Check sheet for the modelled part. Datum: model origin and axes. Units: mm. Round coordinates to 2 decimals unless told otherwise and drop trailing zeros. Order: outer loops, then holes, each group sorted by start corner. A loop starts at its lowest first (then second) coordinate and runs counter-clockwise, first axis right, second up.
```python
from build123d import *

# Parameters (mm, degrees)
F1_DEPTH = 38.1
F2_DEPTH = 38.1
F4_DEPTH = 38.1
F5_DEPTH = 38.1
F7_DEPTH = 38.1
F8_DEPTH = 38.1


with BuildPart() as f1:
    # F0 (on Front) → F1 (new body)
    with BuildSketch(Plane.XZ):
        Polygon((-19.05, 38.1), (-38.1, 19.05), (-38.1, -19.05), (-19.05, -38.1), (19.05, -38.1), (38.1, -19.05), (38.1, 19.05), (19.05, 38.1), align=None)
    extrude(amount=F1_DEPTH)

    # F0 (on Front) → F2 (join)
    with BuildSketch(Plane.XZ):
        Polygon((-19.05, 38.1), (-38.1, 19.05), (-38.1, -19.05), (-19.05, -38.1), (19.05, -38.1), (38.1, -19.05), (38.1, 19.05), (19.05, 38.1), align=None)
    extrude(amount=-F2_DEPTH)

    # F3 (on Right) → F4 (cut)
    with BuildSketch(Plane.YZ):
        Polygon((-38.1, 38.1), (-38.1, 19.05), (-19.05, 38.1), align=None)
        Polygon((38.1, 38.1), (19.05, 38.1), (38.1, 19.05), align=None)
        Polygon((38.1, -19.05), (19.05, -38.1), (38.1, -38.1), align=None)
        Polygon((-19.05, -38.1), (-38.1, -19.05), (-38.1, -38.1), align=None)
    extrude(amount=-F4_DEPTH, mode=Mode.SUBTRACT)

    # F3 (on Right) → F5 (cut)
    with BuildSketch(Plane.YZ):
        Polygon((-38.1, 38.1), (-38.1, 19.05), (-19.05, 38.1), align=None)
        Polygon((38.1, 38.1), (19.05, 38.1), (38.1, 19.05), align=None)
        Polygon((38.1, -19.05), (19.05, -38.1), (38.1, -38.1), align=None)
        Polygon((-19.05, -38.1), (-38.1, -19.05), (-38.1, -38.1), align=None)
    extrude(amount=F5_DEPTH, mode=Mode.SUBTRACT)

    # F6 (on Top) → F7 (cut)
    with BuildSketch(Plane.XY):
        Polygon((38.1, -19.05), (19.05, -38.1), (38.1, -38.1), align=None)
        Polygon((19.05, 38.1), (38.1, 19.05), (38.1, 38.1), align=None)
        Polygon((-38.1, 38.1), (-38.1, 19.05), (-19.05, 38.1), align=None)
        Polygon((-38.1, -38.1), (-19.05, -38.1), (-38.1, -19.05), align=None)
    extrude(amount=-F7_DEPTH, mode=Mode.SUBTRACT)

    # F6 (on Top) → F8 (cut)
    with BuildSketch(Plane.XY):
        Polygon((38.1, -19.05), (19.05, -38.1), (38.1, -38.1), align=None)
        Polygon((-38.1, -38.1), (-19.05, -38.1), (-38.1, -19.05), align=None)
        Polygon((-38.1, 38.1), (-38.1, 19.05), (-19.05, 38.1), align=None)
        Polygon((19.05, 38.1), (38.1, 19.05), (38.1, 38.1), align=None)
    extrude(amount=F8_DEPTH, mode=Mode.SUBTRACT)


solid = f1.part
```
Item 1: Scan lines: line 1 along Z through (x, y) = (28.5, -9); line 2 along Z through (x, y) = (-20.5, 24); line 3 along X through (y, z) = (21, 34). Record each from-to range of solid material in increasing order.
Answer:
line 1: z = -28.65 to 28.65
line 2: z = -33.15 to 33.15
line 3: x = -23.15 to 23.15
Item 2: Sectioned sample at B-B (y = -25.5). Record the cut outline in (x, z), and give its area (3 significant figures).
Answer:
outline: (-31.65, -25.5) - (-25.5, -31.65) - (25.5, -31.65) - (31.65, -25.5) - (31.65, 25.5) - (25.5, 31.65) - (-25.5, 31.65) - (-31.65, 25.5) - close
area: 3,930 mm2
Item 3: Go/stop test with flat-tipped pins: P1, Ø10, axis at x = 30.5, z = 7, coming from the +Y side; P2, Ø1, axis at x = -20.5, y = -14.5, coming from the -Z side; P3, Ø4, axis at x = -30, z = 11, coming from the +Y side. Record where each tip stops, or that it passes through.
Answer:
P1: stops at y = 31.65
P2: stops at z = -37.15
P3: stops at y = 29.15
Item 4: Sectioned sample at A-A (x = -14). Record the cut outline in (y, z), and give its area (3 significant figures).
Answer:
outline: (-38.1, -19.05) - (-19.05, -38.1) - (19.05, -38.1) - (38.1, -19.05) - (38.1, 19.05) - (19.05, 38.1) - (-19.05, 38.1) - (-38.1, 19.05) - close
area: 5,080 mm2
